Drawing for the job (mm, zero at the part's lowest x, y, z). Give positions to 0.01 mm unless a question says otherwise; leave off trailing zeros. Loops run counter-clockwise (first coordinate to the right, second up) from the corner with the lowest first, then second, coordinate; pieces in that order, holes last. Notation, with made-up numbers: (59.25, 88) -> (90.25, 88) arc R28 ccw to (90.25, 121) -> close; hole circle Ø1 at (55.5, 83). An arc over 180 degrees is marked (long way). Use CSV: the item, a comma, the result in double quotes. Start each with the question number.
(1) Cut at C-C on y = 2.35. Write the cut outline in (x, z).
(2) Cut at A-A on z = 19.18. Write the cut outline in (x, y).
(3) Drill centre lines: probe 1 along X at (y, z) = (2.85, 19.18); probe 2 along X at (y, z) = (3.7, 18.5) (1 decimal); probe 3 along Z at (x, y) = (4.75, 2.5) (1 decimal). Where is each one in solid material? Low to high.
(4) Flat gauge pin, fed straight in: pin 1 (4 mm diameter, centred on x = 9.5, z = 33.5, fed in from -Y). Where does the tip first touch, or does it go through?
(5) Cut at B-B on y = 4.1. State how many separate pieces and enclosed holes the cut face has, then the cut area to 3 significant figures.
(6) Cut at D-D on z = 8.65. Write the cut outline in (x, y).
(7) Pull direction X, two halves, no side cores. Call the marked faces 1, 2 and 3: pulls with the +X half, pulls with the -X half, needs draft (parallel to the pull), parting line crosses it, or undercut.
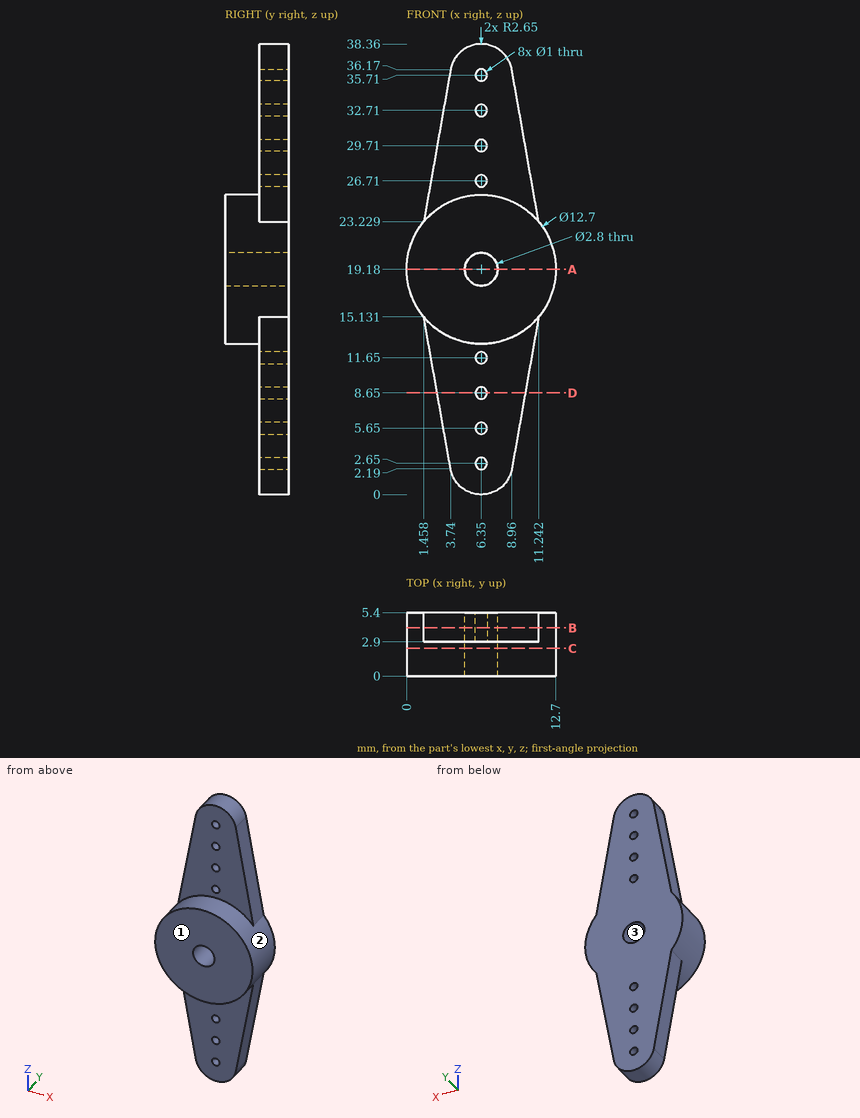
Check result:
1,outline,"circle Ø12.7 at (6.35, 19.18); hole circle Ø2.8 at (6.35, 19.18)"
2,outline,"(0, 0) -> (4.95, 0) -> (4.95, 5.4) -> (0, 5.4) -> close; (7.75, 0) -> (12.7, 0) -> (12.7, 5.4) -> (7.75, 5.4) -> close"
3,probe 1,"0 to 4.95, 7.75 to 12.7"
3,probe 2,"0 to 5.1, 7.6 to 12.7"
3,probe 3,"13 to 25.3"
4,pin 1,"y = 2.9"
5,separate pieces,"1"
5,enclosed holes,"9"
5,area,"294 mm²"
6,outline,"(2.6, 2.9) -> (5.85, 2.9) -> (5.85, 5.4) -> (2.6, 5.4) -> close; (6.85, 2.9) -> (10.1, 2.9) -> (10.1, 5.4) -> (6.85, 5.4) -> close"
7,face 1,"needs draft"
7,face 2,"parting line crosses it"
7,face 3,"undercut"
